The listing builds one solid part. Answer for the finished solid, in the listing's coordinates (mm). A direction names the side the tool comes from. Round coordinates to 2 decimals unless told otherwise and drop trailing zeros. Write each loop counter-clockwise with the first axis right and the second up, starting at its lowest first coordinate (ties: lowest second). Pieces come first, ordered by that corner, then holes.
from build123d import *

# Parameters (mm, degrees)
SKETCH1_W           = 393.7
SKETCH1_H           = 120.65
BOSS_EXTRUDE1_DEPTH = 6.35
CUT_EXTRUDE1_DEPTH  = 7.35


with BuildPart() as part:
    # Sketch1 → Boss-Extrude1 (new body)
    with BuildSketch(Plane.XY):
        with Locations((196.85, 60.325)):
            Rectangle(SKETCH1_W, SKETCH1_H)
    extrude(amount=BOSS_EXTRUDE1_DEPTH)

    # Sketch2 → Cut-Extrude1 (cut, through all)
    with BuildSketch(Plane.XY.offset(6.35)):
        Polygon((133.805909488, 120.65), (177.8, 95.25), (279.4, 95.25), (323.394090512, 120.65), align=None)
        Polygon((133.805909488, 0), (177.8, 25.4), (279.4, 25.4), (323.394090512, 0), align=None)
    extrude(amount=-CUT_EXTRUDE1_DEPTH, mode=Mode.SUBTRACT)


solid = part.part
1. Straight lines are drawn through the part: line 1 along Y through (x, z) = (211, 4.75); line 2 along X through (y, z) = (6, 5.25); line 3 along X through (y, z) = (104, 2). For each, find the intervals that lie inside material, in ascending order.
Geometry says:
line 1: y = 25.4 to 95.25
line 2: x = 0 to 144.2, 313 to 393.7
line 3: x = 0 to 162.64, 294.56 to 393.7
2. A tool of negligible diameter and unlimited length cuts with its end or side. For faces 1 (the face through (155.49, 12.52, 3.22)), 2 (the face through (358, 120.65, 3)), 3 (the face through (301.089, 107.772, 3.219)), from which of +Z, -Z, +X, -X, +Y, -Y can it reach the whole face along a straight path? Write none if from no direction.
Geometry says:
face 1: +Z, -Z, -Y
face 2: +Z, -Z, +X, -X, +Y
face 3: +Z, -Z, +Y
3. Given pin 1 (3 mm diameter, centred on x = 233, z = 1.5, fed in from -Y), flat-ended and moving along its own axis, determine where the tip first touches the part or whether it passes through.
Geometry says:
pin 1: stops at y = 25.4
4. For a pull along X with two mould halves and no side action, classify faces 4 (the face through (194, 61, 6.35)), 5 (the face through (228, 25.4, 3)), 6 (the face through (393.7, 59, 3)) as released by +X, released by -X, zero draft, split by the parting line, or undercut.
Geometry says:
face 4: zero draft
face 5: undercut
face 6: released by +X
5. Section C-C on x = 200 is taken. Determine the outline of the cut face in (y, z), plus the area to 3 significant figures.
Geometry says:
outline: (25.4, 0) - (95.25, 0) - (95.25, 6.35) - (25.4, 6.35) - close
area: 444 mm2
6. Section D-D on y = 112 is taken. Determine the outline of the cut face in (x, z), plus the area to 3 significant figures.
Geometry says:
outline: (0, 0) - (148.79, 0) - (148.79, 6.35) - (0, 6.35) - close; (308.41, 0) - (393.7, 0) - (393.7, 6.35) - (308.41, 6.35) - close
area: 1,490 mm2
7. Section B-B on z = 1.5 is taken. Determine the outline of the cut face in (x, y).
Geometry says:
outline: (0, 0) - (133.81, 0) - (177.8, 25.4) - (279.4, 25.4) - (323.39, 0) - (393.7, 0) - (393.7, 120.65) - (323.39, 120.65) - (279.4, 95.25) - (177.8, 95.25) - (133.81, 120.65) - (0, 120.65) - close
8. Section A-A on y = 20 is taken. Determine the outline of the cut face in (x, z), plus the area to 3 significant figures.
Geometry says:
outline: (0, 0) - (168.45, 0) - (168.45, 6.35) - (0, 6.35) - close; (288.75, 0) - (393.7, 0) - (393.7, 6.35) - (288.75, 6.35) - close
area: 1,740 mm2
